Autodesk Inventor part; units mm, degrees
ref_plane "YZ Plane" through (0, 0, 0) normal (1, 0, 0) x (0, 1, 0)
ref_plane "XZ Plane" through (0, 0, 0) normal (0, 1, 0) x (-1, 0, 0)
ref_plane "XY Plane" through (0, 0, 0) normal (0, 0, 1) x (1, 0, 0)
sketch "スケッチ1" plane through (0, 0, 0) normal (0, 0, 1) x (1, 0, 0)
  circle A0 centre (0, 0) radius 8
  circle A1 centre (0, 0) radius 6
  circle A2 centre (0, 0) radius 1.25
  circle A3 centre (-2.8, -2.8) radius 1.5
  circle A4 centre (-2.8, 2.8) radius 1.5
  circle A5 centre (2.8, 2.8) radius 1.5
  circle A6 centre (2.8, -2.8) radius 1.5
  circle A7 centre (0, 0) radius 6
  dimension "d0" = 16
  dimension "d1" = 12
extrude "押し出し1" add sketch "スケッチ1" along normal blind 4 contours A1
properties part number "新型３脚最終段カム" material "アルミニウム 2014-T4"
The listing builds one solid part. Answer for the finished solid, in the listing's coordinates (mm). Give positions to 0.01 mm unless a question says otherwise; leave off trailing zeros. Write each loop counter-clockwise with the first axis right and the second up, starting at its lowest first coordinate (ties: lowest second). Pieces come first, ordered by that corner, then holes. Notation, with made-up numbers: (31.5, 15.5) -> (49.5, 15.5) arc R18 cw to (49.5, 46.5) -> close; hole circle Ø11 at (35.25, -2.75). An arc over 180 degrees is marked (long way). One line per question, with ' | ' between items. Start each with the question number.
1. Find the intervals of material crossed by probe 1 along Y at (x, z) = (-2.75, 2.05); probe 2 along Y at (x, z) = (-4, 0.4); probe 3 along Y at (x, z) = (0, 1), in increasing order.
2. Section A-A (x = 0) is taken. Determine the outline of the cut face in (y, z), plus the area to 3 significant figures.
3. Section C-C (y = 2.8) is taken. Determine the outline of the cut face in (x, z), plus the area to 3 significant figures.
4. Given pin 1 Ø1 at (x, z) = (-4, 2.5) entering from +Y; pin 2 Ø1.5 at (x, z) = (3.5, 3.5) entering from -Y, each flat-ended and moving along its own axis, determine where each tip first touches the part or whether it passes through.
5. Section D-D (x = -1.75) is taken. Determine the outline of the cut face in (y, z).
6. Section B-B (z = 2.8) is taken. Determine the outline of the cut face in (x, y), plus the area to 3 significant figures.
7. For a pull along X with two mould halves and no side action, classify faces 1 (the cylindrical face through (-6, 0, 2)), 2 (the cylindrical face through (-3.91, 1.79, 1.97)), 3 (the flat face through (1, -1, 4)) as pulls with the +X half, pulls with the -X half, needs draft (parallel to the pull), parting line crosses it, or undercut.
Response values:
1) probe 1: -5.33 to -4.3, -1.3 to 1.3, 4.3 to 5.33 | probe 2: -4.47 to -3.7, -1.9 to 1.9, 3.7 to 4.47 | probe 3: -6 to -1.25, 1.25 to 6
2) outline: (-6, 0) -> (-1.25, 0) -> (-1.25, 4) -> (-6, 4) -> close; (1.25, 0) -> (6, 0) -> (6, 4) -> (1.25, 4) -> close | area: 38.0 mm2
3) outline: (-5.31, 0) -> (-4.3, 0) -> (-4.3, 4) -> (-5.31, 4) -> close; (-1.3, 0) -> (1.3, 0) -> (1.3, 4) -> (-1.3, 4) -> close; (4.3, 0) -> (5.31, 0) -> (5.31, 4) -> (4.3, 4) -> close | area: 18.5 mm2
4) pin 1: y = 4.87 | pin 2: y = -5.33
5) outline: (-5.74, 0) -> (-3.87, 0) -> (-3.87, 4) -> (-5.74, 4) -> close; (-1.73, 0) -> (1.73, 0) -> (1.73, 4) -> (-1.73, 4) -> close; (3.87, 0) -> (5.74, 0) -> (5.74, 4) -> (3.87, 4) -> close
6) outline: circle Ø12 at (0, 0); hole circle Ø3 at (-2.8, -2.8); hole circle Ø3 at (-2.8, 2.8); hole circle Ø2.5 at (0, 0); hole circle Ø3 at (2.8, -2.8); hole circle Ø3 at (2.8, 2.8) | area: 79.9 mm2
7) face 1: parting line crosses it | face 2: undercut | face 3: needs draft
